Geometry: final body of the model. Coordinates: model frame, mm. Face numbers are marked on the shaded views. A direction names the side the tool comes from. Give positions to 0.01 mm unless a question says otherwise; leave off trailing zeros. Order: outer loops, then holes, each group sorted by start corner. A loop starts at its lowest first (then second) coordinate and runs counter-clockwise, first axis right, second up. Notation, with made-up numbers: (60, 68.25) -> (99, 68.25) arc R22 ccw to (99, 75.25) -> close; hole circle Ø8 at (-6, -23.75). An arc over 180 degrees is marked (long way). Answer in a Markdown table with one row per item. Add a question column.
Q1. Contact query for flat-ended pins moving along their axis: P1, Ø4, axis at x = -12, y = -19.5, coming from the -Z side; P2, Ø10, axis at y = -5.5, z = -12, coming from the +X side; P3, Ø1, axis at y = -14, z = -14.5, coming from the -X side. Output: stop coordinate, or through.
Q2. Pull-direction query (Z, two-part tool) for the marked faces 1, 2, 3 and 4; classes: +Z half, -Z half, draft (parallel to the pull), parting line (faces both ways), or undercut.
Q3. Cut plane B-B on z = 2.5. Return the cut outline in (x, y).
Q4. Cut plane C-C on x = 4.5. Return the cut outline in (y, z), and give its area (3 significant figures).
Q5. Cut plane A-A on z = 8.5. Return the cut outline in (x, y).
Q6. Set-up query: the marked faces 5, 6 and 7. Return all of +Z, -Z, +X, -X, +Y, -Y with unobstructed straight access to the full face (end or side cutting, diameter ignored); none if empty.
Q7. Line query: line 1 along X through (y, z) = (-21.5, -12); line 2 along X through (y, z) = (-22, 6); line 3 along X through (y, z) = (-6, 4). Output: solid intervals per line, ascending. Write a range as from..to.
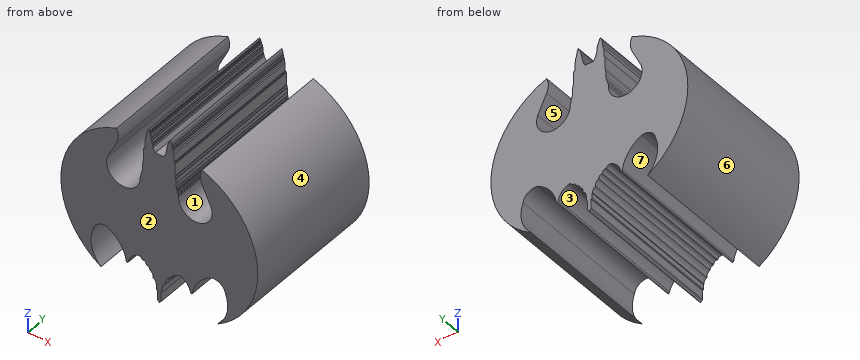
from build123d import *

# Parameters (mm, degrees)
F1_DEPTH = 25.4


with BuildPart() as f1:
    # F0 (on Front) → F1 (new body)
    with BuildSketch(Plane.XZ):
        with BuildLine():
            ThreePointArc((11.683757, -9.757952), (11.910295, -13.005869), (10.289053, -15.829317))
            ThreePointArc((10.289053, -15.829317), (17.279713, -1.751364), (7.521968, 10.571157))
            ThreePointArc((7.521968, 10.571157), (7.225303, 9.272076), (7.521968, 7.972996))
            Line((7.521968, 7.972996), (9.089584, 4.719736))
            ThreePointArc((9.089584, 4.719736), (6.917131, 0.708181), (3.376378, 3.584845))
            Line((3.376378, 3.584845), (3.376378, 3.804322))
            Line((3.376378, 3.804322), (3.344805, 3.804322))
            Line((3.344805, 3.804322), (3.344805, 4.047158))
            Line((3.344805, 4.047158), (3.268356, 4.047158))
            Line((3.268356, 4.047158), (3.268356, 4.348455))
            Line((3.268356, 4.348455), (3.218889, 4.348455))
            Line((3.218889, 4.348455), (3.218889, 4.654248))
            Line((3.218889, 4.654248), (3.110962, 4.654248))
            Line((3.110962, 4.654248), (3.110962, 4.8746))
            Line((3.110962, 4.8746), (3.052502, 4.8746))
            Line((3.052502, 4.8746), (3.052502, 5.247848))
            Line((3.052502, 5.247848), (2.98055, 5.247848))
            Line((2.98055, 5.247848), (2.98055, 5.855694))
            Line((2.98055, 5.855694), (2.941553, 5.855694))
            Line((2.941553, 5.855694), (2.941553, 6.657867))
            Line((2.941553, 6.657867), (2.855988, 6.657867))
            Line((2.855988, 6.657867), (2.855988, 7.089451))
            Line((2.855988, 7.089451), (2.765684, 7.089451))
            Line((2.765684, 7.089451), (2.765684, 7.641547))
            Line((2.765684, 7.641547), (2.765684, 9.285447))
            Line((2.765684, 9.285447), (2.69841, 9.285447))
            Line((2.69841, 9.285447), (2.69841, 9.501676))
            Line((2.69841, 9.501676), (2.564857, 9.501676))
            Line((2.564857, 9.501676), (2.564857, 10.264836))
            Line((2.564857, 10.264836), (2.564857, 10.934666))
            Line((2.564857, 10.934666), (2.42448, 11.120381))
            Line((2.42448, 11.120381), (2.42448, 11.597059))
            Line((2.42448, 11.597059), (2.352529, 11.597059))
            Line((2.352529, 11.597059), (2.352529, 11.857883))
            Line((2.352529, 11.857883), (2.280578, 11.857883))
            Line((2.280578, 11.857883), (2.280578, 12.235628))
            Line((2.280578, 12.235628), (2.199632, 12.235628))
            Line((2.199632, 12.235628), (2.199632, 12.451482))
            Line((2.199632, 12.451482), (2.199632, 12.604379))
            Line((2.199632, 12.604379), (2.12768, 12.793251))
            Line((2.12768, 12.793251), (1.947802, 13.197979))
            Line((1.947802, 13.197979), (1.875851, 13.072063))
            Line((1.875851, 13.072063), (1.785911, 12.946148))
            Line((1.785911, 12.946148), (1.785911, 12.757276))
            Line((1.785911, 12.757276), (1.686978, 12.757276))
            Line((1.686978, 12.757276), (1.686978, 12.559409))
            Line((1.686978, 12.559409), (1.588045, 12.559409))
            Line((1.588045, 12.559409), (1.588045, 12.30758))
            Line((1.588045, 12.30758), (1.46213, 12.17267))
            Line((1.46213, 12.17267), (1.46213, 11.839896))
            Line((1.46213, 11.839896), (1.381184, 11.839896))
            Line((1.381184, 11.839896), (1.381184, 11.453156))
            Line((1.381184, 11.453156), (1.318227, 11.453156))
            Line((1.318227, 11.453156), (1.318227, 10.934666))
            Line((1.318227, 10.934666), (1.228288, 10.934666))
            Line((1.228288, 10.934666), (1.228288, 10.66169))
            Line((1.228288, 10.66169), (1.147342, 10.66169))
            Line((1.147342, 10.66169), (1.147342, 10.264836))
            Line((1.147342, 10.264836), (0.697646, 9.573425))
            Line((0.697646, 9.573425), (0, 9.573425))
            Line((0, 9.573425), (-0.697646, 9.573425))
            Line((-0.697646, 9.573425), (-1.147342, 10.264836))
            Line((-1.147342, 10.264836), (-1.147342, 10.66169))
            Line((-1.147342, 10.66169), (-1.228288, 10.66169))
            Line((-1.228288, 10.66169), (-1.228288, 10.934666))
            Line((-1.228288, 10.934666), (-1.318227, 10.934666))
            Line((-1.318227, 10.934666), (-1.318227, 11.453156))
            Line((-1.318227, 11.453156), (-1.381184, 11.453156))
            Line((-1.381184, 11.453156), (-1.381184, 11.839896))
            Line((-1.381184, 11.839896), (-1.46213, 11.839896))
            Line((-1.46213, 11.839896), (-1.46213, 12.17267))
            Line((-1.46213, 12.17267), (-1.588045, 12.30758))
            Line((-1.588045, 12.30758), (-1.588045, 12.559409))
            Line((-1.588045, 12.559409), (-1.686978, 12.559409))
            Line((-1.686978, 12.559409), (-1.686978, 12.757276))
            Line((-1.686978, 12.757276), (-1.785911, 12.757276))
            Line((-1.785911, 12.757276), (-1.785911, 12.946148))
            Line((-1.785911, 12.946148), (-1.875851, 13.072063))
            Line((-1.875851, 13.072063), (-1.947802, 13.197979))
            Line((-1.947802, 13.197979), (-2.12768, 12.793251))
            Line((-2.12768, 12.793251), (-2.199632, 12.604379))
            Line((-2.199632, 12.604379), (-2.199632, 12.451482))
            Line((-2.199632, 12.451482), (-2.199632, 12.235628))
            Line((-2.199632, 12.235628), (-2.280578, 12.235628))
            Line((-2.280578, 12.235628), (-2.280578, 11.857883))
            Line((-2.280578, 11.857883), (-2.352529, 11.857883))
            Line((-2.352529, 11.857883), (-2.352529, 11.597059))
            Line((-2.352529, 11.597059), (-2.42448, 11.597059))
            Line((-2.42448, 11.597059), (-2.42448, 11.120381))
            Line((-2.42448, 11.120381), (-2.564857, 10.934666))
            Line((-2.564857, 10.934666), (-2.564857, 10.264836))
            Line((-2.564857, 10.264836), (-2.564857, 9.501676))
            Line((-2.564857, 9.501676), (-2.69841, 9.501676))
            Line((-2.69841, 9.501676), (-2.69841, 9.285447))
            Line((-2.69841, 9.285447), (-2.765684, 9.285447))
            Line((-2.765684, 9.285447), (-2.765684, 7.641547))
            Line((-2.765684, 7.641547), (-2.765684, 7.089451))
            Line((-2.765684, 7.089451), (-2.855988, 7.089451))
            Line((-2.855988, 7.089451), (-2.855988, 6.657867))
            Line((-2.855988, 6.657867), (-2.941553, 6.657867))
            Line((-2.941553, 6.657867), (-2.941553, 5.855694))
            Line((-2.941553, 5.855694), (-2.98055, 5.855694))
            Line((-2.98055, 5.855694), (-2.98055, 5.247848))
            Line((-2.98055, 5.247848), (-3.052502, 5.247848))
            Line((-3.052502, 5.247848), (-3.052502, 4.8746))
            Line((-3.052502, 4.8746), (-3.110962, 4.8746))
            Line((-3.110962, 4.8746), (-3.110962, 4.654248))
            Line((-3.110962, 4.654248), (-3.218889, 4.654248))
            Line((-3.218889, 4.654248), (-3.218889, 4.348455))
            Line((-3.218889, 4.348455), (-3.268356, 4.348455))
            Line((-3.268356, 4.348455), (-3.268356, 4.047158))
            Line((-3.268356, 4.047158), (-3.344805, 4.047158))
            Line((-3.344805, 4.047158), (-3.344805, 3.804322))
            Line((-3.344805, 3.804322), (-3.376378, 3.804322))
            Line((-3.376378, 3.804322), (-3.376378, 3.584845))
            ThreePointArc((-3.376378, 3.584845), (-6.917131, 0.708181), (-9.089584, 4.719736))
            Line((-9.089584, 4.719736), (-7.521968, 7.972996))
            ThreePointArc((-7.521968, 7.972996), (-7.225303, 9.272076), (-7.521968, 10.571157))
            ThreePointArc((-7.521968, 10.571157), (-17.279713, -1.751364), (-10.289053, -15.829317))
            ThreePointArc((-10.289053, -15.829317), (-11.910295, -13.005869), (-11.683757, -9.757952))
            ThreePointArc((-11.683757, -9.757952), (-10.801152, -8.348372), (-9.162284, -8.065494))
            ThreePointArc((-9.162284, -8.065494), (-6.955625, -9.887781), (-5.836201, -12.521592))
            ThreePointArc((-5.836201, -12.521592), (-5.616042, -12.688557), (-5.483937, -12.445873))
            ThreePointArc((-5.483937, -12.445873), (-4.875184, -11.247178), (-3.772633, -10.477873))
            ThreePointArc((-3.772633, -10.477873), (-3.293187, -10.529047), (-2.987732, -10.902121))
            ThreePointArc((-2.987732, -10.902121), (-2.478858, -11.006497), (-2.304193, -11.49572))
            ThreePointArc((-2.304193, -11.49572), (-1.83181, -11.65766), (-1.65663, -12.125296))
            ThreePointArc((-1.65663, -12.125296), (-1.189071, -12.556765), (-1.099007, -13.186579))
            ThreePointArc((-1.099007, -13.186579), (-0.677638, -13.56305), (-0.591807, -14.121543))
            Line((-0.591807, -14.121543), (-0.484851, -14.121543))
            Line((-0.484851, -14.121543), (-0.484851, -15.041369))
            Line((-0.484851, -15.041369), (-0.335112, -15.13763))
            Line((-0.335112, -15.13763), (-0.335112, -16.196499))
            Line((-0.335112, -16.196499), (-0.335112, -16.755452))
            Line((-0.335112, -16.755452), (-0.192083, -16.906712))
            Line((-0.192083, -16.906712), (0, -17.118476))
            Line((0, -17.118476), (0.192083, -16.906712))
            Line((0.192083, -16.906712), (0.335112, -16.755452))
            Line((0.335112, -16.755452), (0.335112, -16.196499))
            Line((0.335112, -16.196499), (0.335112, -15.13763))
            Line((0.335112, -15.13763), (0.484851, -15.041369))
            Line((0.484851, -15.041369), (0.484851, -14.121543))
            Line((0.484851, -14.121543), (0.591807, -14.121543))
            ThreePointArc((0.591807, -14.121543), (0.677638, -13.56305), (1.099007, -13.186579))
            ThreePointArc((1.099007, -13.186579), (1.189071, -12.556765), (1.65663, -12.125296))
            ThreePointArc((1.65663, -12.125296), (1.83181, -11.65766), (2.304193, -11.49572))
            ThreePointArc((2.304193, -11.49572), (2.478858, -11.006497), (2.987732, -10.902121))
            ThreePointArc((2.987732, -10.902121), (3.293187, -10.529047), (3.772633, -10.477873))
            ThreePointArc((3.772633, -10.477873), (4.875184, -11.247178), (5.483937, -12.445873))
            ThreePointArc((5.483937, -12.445873), (5.616042, -12.688557), (5.836201, -12.521592))
            ThreePointArc((5.836201, -12.521592), (6.955625, -9.887781), (9.162284, -8.065494))
            ThreePointArc((9.162284, -8.065494), (10.801152, -8.348372), (11.683757, -9.757952))
        make_face()
    extrude(amount=F1_DEPTH)


solid = f1.part
Completed:
| question | item | result |
|---|---|---|
| 1 | P1 | stops at z = -15.83 |
| 1 | P2 | stops at x = 16.88 |
| 1 | P3 | stops at x = -12.71 |
| 2 | face 1 | undercut |
| 2 | face 2 | draft |
| 2 | face 3 | -Z half |
| 2 | face 4 | parting line |
| 3 | outline | (-16.17, -25.4) -> (-9.09, -25.4) -> (-9.09, 0) -> (-16.17, 0) -> close; (-3.59, -25.4) -> (3.59, -25.4) -> (3.59, 0) -> (-3.59, 0) -> close; (9.09, -25.4) -> (16.17, -25.4) -> (16.17, 0) -> (9.09, 0) -> close |
| 4 | outline | (-25.4, -10.89) -> (0, -10.89) -> (0, 1.29) -> (-25.4, 1.29) -> close |
| 4 | area | 309 mm² |
| 5 | outline | (-11.43, -25.4) -> (-7.33, -25.4) -> (-7.33, 0) -> (-11.43, 0) -> close; (-2.77, -25.4) -> (2.77, -25.4) -> (2.77, 0) -> (-2.77, 0) -> close; (7.33, -25.4) -> (11.43, -25.4) -> (11.43, 0) -> (7.33, 0) -> close |
| 6 | face 5 | +Y, -Y |
| 6 | face 6 | -X, +Y, -Y |
| 6 | face 7 | -Z, +Y, -Y |
| 7 | line 1 | x = -14.49..-12.05, -5.95..-5.34, -1.66..1.66, 5.34..5.95, 12.05..14.49 |
| 7 | line 2 | x = -14.05..-8.47, -2.94..2.94, 8.47..14.05 |
| 7 | line 3 | x = -15.43..-9.28, -3.34..3.34, 9.28..15.43 |
